Check sheet for the modelled part. Datum: model origin and axes. Units: mm. A direction names the side the tool comes from. Coordinates: 2 decimals unless noted, no trailing zeros. Write each loop counter-clockwise with the first axis right and the second up, starting at its lowest first coordinate (ties: lowest second). Pieces come first, ordered by that corner, then holes. Notation, with made-up numbers: (45.5, 80.5) - (76.5, 80.5) arc R10 cw to (76.5, 96.5) - close; hole circle Ø4 at (63.25, -36). An arc over 180 degrees is marked (long way). Write each question's results on one line, items separated by ' | '.
from build123d import *

# Parameters (mm, degrees)
F0_R     = 26.2810947886
F0_R_2   = 10.298862613
F1_DEPTH = 50.8
F3_T     = -2.54


# Not quite as in the source:
# - a fillet or chamfer that OpenCascade refuses, or shapes differently, is made with other operations: its cross-section is extruded or revolved along the edge and cut away or added


with BuildPart() as f1:
    # F0 (on Front) → F1 (new body)
    with BuildSketch(Plane.XZ):
        Circle(F0_R)
        Circle(F0_R_2, mode=Mode.SUBTRACT)
    extrude(amount=F1_DEPTH)

    # F2: fillet of radius 19.622727835 on 1 edges, made by hand

    # F2_s1 → F2_t2 (revolve, cut)
    with BuildSketch(Plane.XY):
        with BuildLine():
            ThreePointArc((26.2810947886, -31.5179295967), (21.7661117091, -44.0402095843), (10.298862613, -50.8))
            Line((10.298862613, -50.8), (26.2810947886, -50.8))
            Line((26.2810947886, -50.8), (26.2810947886, -31.5179295967))
        make_face()
    revolve(axis=Axis((0, -50.8, 0), (0, -1, 0)), mode=Mode.SUBTRACT)

    # F3
    f3_openings = [f1.faces().sort_by_distance(p)[0] for p in [
        (-10.298863, -25.4, 0),
    ]]
    offset(amount=F3_T, openings=f3_openings)


solid = f1.part
1. Go/stop test with flat-tipped pins: pin 1 (6 mm diameter, centred on x = -12.5, z = -5, fed in from -Y); pin 2 (12 mm diameter, centred on y = -17.5, z = 18, fed in from -X); pin 3 (1.5 mm diameter, centred on x = -6.5, y = -33.5, fed in from -Z). Record where each tip stops, or that it passes through.
Values follow:
pin 1: stops at y = -50.77 | pin 2: stops at x = -23.38 | pin 3: stops at z = -25.56
2. Access from +Z, -Z, +X, -X, +Y, -Y to the whole of each face (thin tool, end or side, straight path). Record for faces 4 (the flat face through (10, -2.54, -5)), 5 (the cylindrical face through (9.823, -49.486, 3.093)).
Values follow:
face 4: none | face 5: +Y, -Y
3. Draft check along Y on faces 1 (the cylindrical face through (-2.233, -1.252, -10.054)), 2 (the flat face through (11, 0, 0)), 3 (the cylindrical face through (22.645, -16.826, 7.131)). Enter one of: pulls with the +Y half, pulls with the -Y half, needs draft (parallel to the pull), parting line crosses it, or undercut.
Values follow:
face 1: needs draft | face 2: pulls with the +Y half | face 3: undercut
4. Sectioned sample at A-A (y = -29). Record the cut outline in (x, z), then the cut area to 3 significant figures.
Values follow:
outline: circle Ø52.56 at (0, 0); hole circle Ø47.48 at (0, 0) | area: 399 mm^2
5. Material ranges on L1, parallel to Z at x = 0, y = -15; L2, parallel to Z at x = 0, y = -2; L3, parallel to X at y = -8.5, z = 16.5, recorded low to high. Write a range as [from, to].
Values follow:
L1: z = [-26.28, -23.74], [23.74, 26.28] | L2: z = [-26.28, -10.3], [10.3, 26.28] | L3: x = [-20.46, -17.07], [17.07, 20.46]
